Job drawing, mm, ordinate dimensions from the low corner. One solid piece. A direction names the side the tool comes from. Give positions to 0.01 mm unless a question says otherwise; leave off trailing zeros. Write each loop counter-clockwise with the first axis right and the second up, starting at its lowest first coordinate (ties: lowest second). Pieces come first, ordered by that corner, then holes. Notation, with made-up numbers: M 14.25,-23.5 L 65.25,-23.5 A16 ccw 65.25,0.5 Z; hole C 55.25,72 d3. An arc over 180 degrees is marked long. Answer as CSV lines item,"result". Start each with the question number.
1) Slice it at D-D, the plane z = 31. Give the cut face in (x, y).
2) Mould opens along X. For the marked faces 1, 2 and 3 say: pulls with the +X half, pulls with the -X half, needs draft (parallel to the pull), parting line crosses it, or undercut.
3) Slice it at A-A, the plane y = 14.25. Give the cut face in (x, z), plus the area to 3 significant figures.
4) Slice it at C-C, the plane x = 9.5. Give the cut face in (y, z), plus the area to 3 significant figures.
5) Tool access for the marked faces 4 and 5: list every direction of +Z, -Z, +X, -X, +Y, -Y with a clear straight run to the whole face (end or side of a thin tool).
6) Pin check, flat tips, straight feed: pin 1 Ø5 at (x, z) = (17, 7) entering from +Y; pin 2 Ø5 at (x, z) = (15, 29.5) entering from +Y. Stop position of each tip, or through.
7) Slice it at B-B, the plane z = 7. Give the cut face in (x, y).
8) Wall check: line 1 along X through (y, z) = (1.2, 27); line 2 along X through (y, z) = (11.25, 12.5); line 3 along Y through (x, z) = (27, 29.5). Give the ranges that are in metal, low to high. Write a range as from..to.
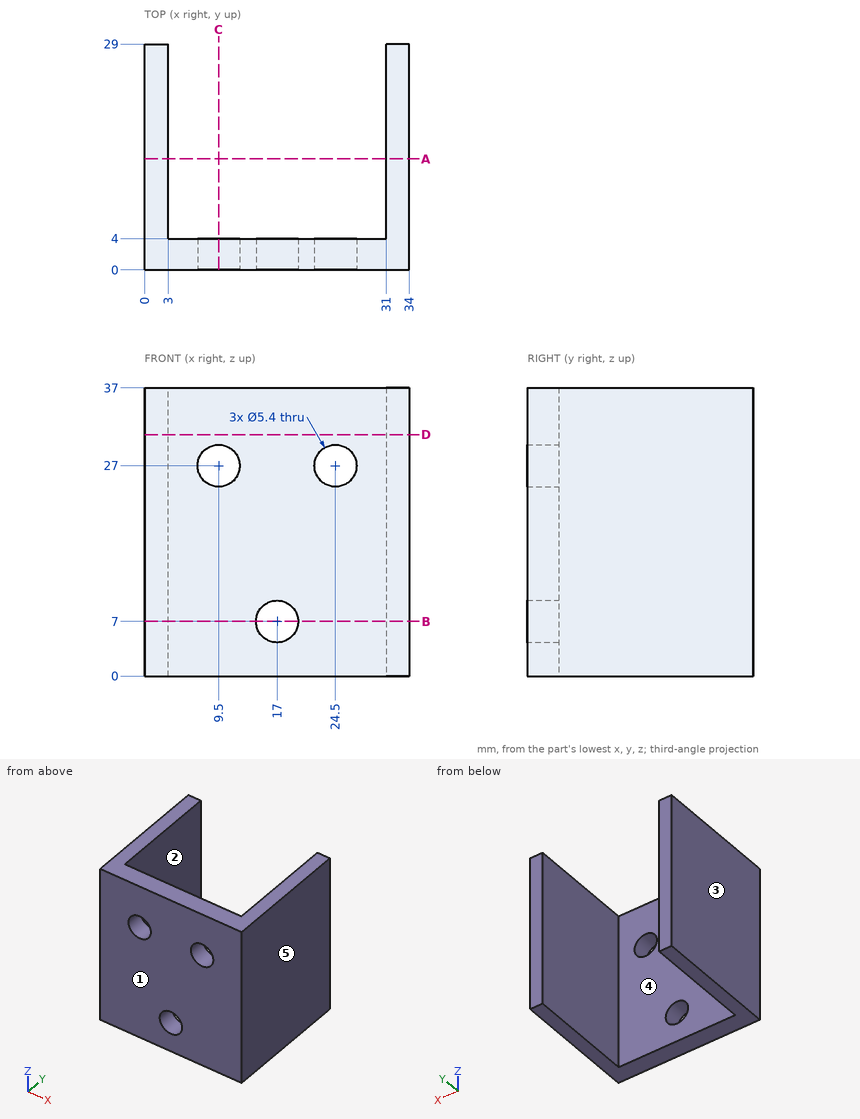
Found:
1,outline,"M 0,0 L 34,0 L 34,29 L 31,29 L 31,4 L 3,4 L 3,29 L 0,29 Z"
2,face 1,"needs draft"
2,face 2,"undercut"
2,face 3,"pulls with the -X half"
3,outline,"M 0,0 L 3,0 L 3,37 L 0,37 Z; M 31,0 L 34,0 L 34,37 L 31,37 Z"
3,area,"222 mm²"
4,outline,"M 0,0 L 4,0 L 4,24.3 L 0,24.3 Z; M 0,29.7 L 4,29.7 L 4,37 L 0,37 Z"
4,area,"126 mm²"
5,face 4,"+Z, -Z, +Y"
5,face 5,"+Z, -Z, +X, +Y, -Y"
6,pin 1,"through"
6,pin 2,"y = 4"
7,outline,"M 0,0 L 14.3,0 L 14.3,4 L 3,4 L 3,29 L 0,29 Z; M 19.7,0 L 34,0 L 34,29 L 31,29 L 31,4 L 19.7,4 Z"
8,line 1,"0..6.8, 12.2..21.8, 27.2..34"
8,line 2,"0..3, 31..34"
8,line 3,"0..4"
